from build123d import *

# Parameters (mm, degrees)
SKETCH1_W               = 100
SKETCH1_H               = 50
BOSS_EXTRUDE1_DEPTH     = 10
SKETCH2_W               = 2.5
SKETCH2_H               = 5
CUT_EXTRUDE1_DEPTH      = 1
CUT_EXTRUDE1_DEPTH_BACK = 101
SKETCH4_W               = 5
SKETCH4_H               = 30
BOSS_EXTRUDE2_DEPTH     = 80
SKETCH5_R               = 3.173204402
CUT_EXTRUDE3_DEPTH      = 21
CUT_EXTRUDE3_DEPTH_BACK = 81
FILLET1_R               = 10
FILLET2_R               = 10


with BuildPart() as part:
    # Sketch1 → Boss-Extrude1 (new body)
    with BuildSketch(Plane.XY):
        with Locations((50, 25)):
            Rectangle(SKETCH1_W, SKETCH1_H)
    extrude(amount=BOSS_EXTRUDE1_DEPTH)

    # Sketch2 → Cut-Extrude1 (cut, two sides)
    with BuildSketch(Plane.ZY) as cut_extrude1_sk:
        with Locations((1.25, 42.5)):
            Rectangle(SKETCH2_W, SKETCH2_H)
        with Locations((1.25, 7.5)):
            Rectangle(SKETCH2_W, SKETCH2_H)
    extrude(amount=CUT_EXTRUDE1_DEPTH, mode=Mode.SUBTRACT)
    extrude(cut_extrude1_sk.sketch, amount=-CUT_EXTRUDE1_DEPTH_BACK, mode=Mode.SUBTRACT)

    # Sketch4 → Boss-Extrude2 (add)
    with BuildSketch(Plane(origin=(0, 0, 0), x_dir=(-1, 0, 0), z_dir=(0, 0, -1))):
        with Locations((-77.5, 25)):
            Rectangle(SKETCH4_W, SKETCH4_H)
        with Locations((-22.5, 25)):
            Rectangle(SKETCH4_W, SKETCH4_H)
    extrude(amount=BOSS_EXTRUDE2_DEPTH)

    # Sketch5 → Cut-Extrude3 (cut, two sides)
    with BuildSketch(Plane(origin=(80, 0, 0), x_dir=(0, 0, -1), z_dir=(1, 0, 0))) as cut_extrude3_sk:
        with Locations((60, 25)):
            Circle(SKETCH5_R)
    extrude(amount=CUT_EXTRUDE3_DEPTH, mode=Mode.SUBTRACT)
    extrude(cut_extrude3_sk.sketch, amount=-CUT_EXTRUDE3_DEPTH_BACK, mode=Mode.SUBTRACT)

    # Fillet1
    fillet1_edges = [part.edges().sort_by_distance(p)[0] for p in [
        (77.5, 40, -80),
        (77.5, 10, -80),
        (22.5, 10, -80),
        (22.5, 40, -80),
    ]]
    fillet(fillet1_edges, radius=FILLET1_R)

    # Fillet2
    fillet2_edges = [part.edges().sort_by_distance(p)[0] for p in [
        (80, 25, 0),
        (20, 25, 0),
    ]]
    fillet(fillet2_edges, radius=FILLET2_R)


solid = part.part
The listing builds one solid part. Answer for the finished solid, in the listing's coordinates (mm). A direction names the side the tool comes from. Coordinates: 2 decimals unless noted, no trailing zeros. Loops run counter-clockwise (first coordinate to the right, second up) from the corner with the lowest first, then second, coordinate; pieces in that order, holes last.
1) Find section A-A on y = 25. Write down the section's boundary in (x, z).
2) Determine the mould class of faces 6 (the face through (22.535, 25.953, -63.027)), 7 (the face through (25, 25, -39)), 8 (the face through (49, 50, 5)) for opening direction Y: pulls with the +Y half, pulls with the -Y half, needs draft (parallel to the pull), parting line crosses it, or undercut.
3) Find section B-B on z = -31. Write down the section's boundary in (x, y).
4) Find section C-C on z = -60. Write down the section's boundary in (x, y).
5) Flat-ended cylindrical pins translate along their axes: pin 1 Ø3 at (x, y) = (97.5, 21.5) entering from -Z; pin 2 Ø15 at (y, z) = (23, -48.5) entering from -X; pin 3 Ø1.5 at (y, z) = (32, -52) entering from +X. Find the tip coordinate at first contact, or state that the pin passes through.
6) Find section D-D on x = 93. Write down the section's boundary in (y, z), then the cut area to 3 significant figures.
7) Find the intervals of material crossed by L1, parallel to Y at x = 23.4, z = -60; L2, parallel to X at y = 11.5, z = -45; L3, parallel to Z at x = 67.5, y = 41, in increasing order.
8) A tool of negligible diameter and unlimited length cuts with its end or side. For faces 1 (the face through (95, 25, 0)), 2 (the face through (49, 42, 2.5)), 3 (the face through (20, 25, -45)), 4 (the face through (49, 3, 0)), 5 (the face through (75, 25, -39)), from which of +Z, -Z, +X, -X, +Y, -Y can it reach the whole face along a straight path? Write none if from no direction.
Values:
1. outline: (0, 0) - (10, 0) arc R10 cw to (20, -10) - (20, -56.83) - (25, -56.83) - (25, 0) - (75, 0) - (75, -56.83) - (80, -56.83) - (80, -10) arc R10 cw to (90, 0) - (100, 0) - (100, 10) - (0, 10) - close; (20, -80) - (25, -80) - (25, -63.17) - (20, -63.17) - close; (75, -80) - (80, -80) - (80, -63.17) - (75, -63.17) - close
2. face 6: undercut
2. face 7: needs draft
2. face 8: pulls with the +Y half
3. outline: (20, 10) - (25, 10) - (25, 40) - (20, 40) - close; (75, 10) - (80, 10) - (80, 40) - (75, 40) - close
4. outline: (20, 10) - (25, 10) - (25, 21.83) - (20, 21.83) - close; (20, 28.17) - (25, 28.17) - (25, 40) - (20, 40) - close; (75, 10) - (80, 10) - (80, 21.83) - (75, 21.83) - close; (75, 28.17) - (80, 28.17) - (80, 40) - (75, 40) - close
5. pin 1: stops at z = 0
5. pin 2: stops at x = 20
5. pin 3: stops at x = 80
6. outline: (0, 0) - (5, 0) - (5, 2.5) - (10, 2.5) - (10, 0) - (40, 0) - (40, 2.5) - (45, 2.5) - (45, 0) - (50, 0) - (50, 10) - (0, 10) - close
6. area: 475 mm2
7. L1: y = 10 to 21.83, 28.17 to 40
7. L2: x = 20 to 25, 75 to 80
7. L3: z = 2.5 to 10
8. face 1: -Z, +X, +Y, -Y
8. face 2: -Z, +X, -X
8. face 3: -Z, -X, +Y, -Y
8. face 4: -Z, +X, -X, -Y
8. face 5: -Z, +Y, -Y
